from build123d import *

# Parameters (mm, degrees)
SKETCH1_W               = 30
SKETCH1_H               = 15
BOSS_EXTRUDE1_DEPTH     = 30
CUT_EXTRUDE1_DEPTH      = 35.369317712
CUT_EXTRUDE1_DEPTH_BACK = 35.369317712
SKETCH2_R               = 2.75
SKETCH3_R               = 4.75
CUT_EXTRUDE3_DEPTH      = 5.5


with BuildPart() as part:
    # Sketch1 → Boss-Extrude1 (new body)
    with BuildSketch(Plane(origin=(0, 0, 0), x_dir=(1, 0, 0), z_dir=(0, 1, 0))):
        Rectangle(SKETCH1_W, SKETCH1_H)
    extrude(amount=BOSS_EXTRUDE1_DEPTH)

    # Sketch2 → Cut-Extrude1 (cut, two sides: drawn at the far end of the back side and taken through both)
    with BuildSketch(Plane(origin=(0, 0, 0), x_dir=(1, 0, 0), z_dir=(0, 1, 0)).offset(-CUT_EXTRUDE1_DEPTH_BACK)):
        with Locations(Location((0, 0, 0), (0, 0, 270))):
            Circle(SKETCH2_R)
    extrude(amount=CUT_EXTRUDE1_DEPTH + CUT_EXTRUDE1_DEPTH_BACK, mode=Mode.SUBTRACT)

    # Sketch3 → Cut-Extrude3 (cut)
    with BuildSketch(Plane(origin=(0, 30, 0), x_dir=(1, 0, 0), z_dir=(0, 1, 0))):
        with Locations(Location((0, 0, 0), (0, 0, 270))):
            Circle(SKETCH3_R)
    extrude(amount=-CUT_EXTRUDE3_DEPTH, mode=Mode.SUBTRACT)


solid = part.part
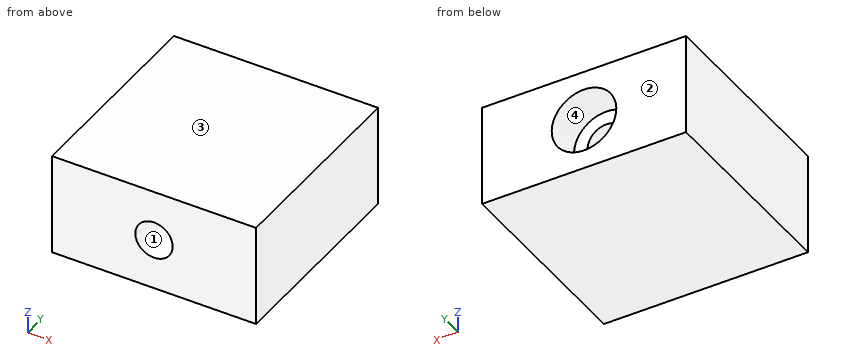
Verification items for the finished model (mm, model axes). Face numbers are marked on the shaded views. Round coordinates to 2 decimals unless told otherwise and drop trailing zeros. Order: outer loops, then holes, each group sorted by start corner. A loop starts at its lowest first (then second) coordinate and runs counter-clockwise, first axis right, second up. Notation, with made-up numbers: (43.25, 2) -> (62.25, 2) arc R25 ccw to (62.25, 36) -> close; hole circle Ø6 at (33.5, -18.75). An arc over 180 degrees is marked (long way). Put each result on its own line as item: value.
1) Section check A-A (x = 0). Record the cut outline in (y, z).
Final values:
outline: (0, -7.5) -> (30, -7.5) -> (30, -4.75) -> (24.5, -4.75) -> (24.5, -2.75) -> (0, -2.75) -> close; (0, 2.75) -> (24.5, 2.75) -> (24.5, 4.75) -> (30, 4.75) -> (30, 7.5) -> (0, 7.5) -> close
2) Section check B-B (z = -2). Record the cut outline in (x, y), then the cut area to 3 significant figures.
Final values:
outline: (-15, 0) -> (-1.89, 0) -> (-1.89, 24.5) -> (-4.31, 24.5) -> (-4.31, 30) -> (-15, 30) -> close; (1.89, 0) -> (15, 0) -> (15, 30) -> (4.31, 30) -> (4.31, 24.5) -> (1.89, 24.5) -> close
area: 760 mm^2
3) Depth check by flat-ended pin: pin 1 (5 mm diameter, centred on x = -4.5, z = 5.5, fed in from -Y). Enter the tip coordinate at first touch or a pass-through.
Final values:
pin 1: stops at y = 0
4) Material ranges on line 1 (X direction, y = 26.5, z = 0); line 2 (X direction, y = 9.75, z = 0); line 3 (Z direction, x = 0, y = 11.5), recorded low to high.
Final values:
line 1: x = -15 to -4.75, 4.75 to 15
line 2: x = -15 to -2.75, 2.75 to 15
line 3: z = -7.5 to -2.75, 2.75 to 7.5
5) Mould release check, pull along Z, two halves, no side actions. Record for the marked faces 1, 2, 3 and 4: +Z half, -Z half, draft (parallel to the pull), parting line (faces both ways), or undercut.
Final values:
face 1: undercut
face 2: draft
face 3: +Z half
face 4: undercut
6) Section check C-C (y = 19.5). Record the cut outline in (x, z).
Final values:
outline: (-15, -7.5) -> (15, -7.5) -> (15, 7.5) -> (-15, 7.5) -> close; hole circle Ø5.5 at (0, 0)
7) Section check D-D (z = -4). Record the cut outline in (x, y), then the cut area to 3 significant figures.
Final values:
outline: (-15, 0) -> (15, 0) -> (15, 30) -> (2.56, 30) -> (2.56, 24.5) -> (-2.56, 24.5) -> (-2.56, 30) -> (-15, 30) -> close
area: 872 mm^2
